from build123d import *

# Parameters (mm, degrees)
F0_W      = 609.6
F0_H      = 762
F1_DEPTH  = 203.2
F2_W      = 76.2
F2_H      = 609.6
F3_DEPTH  = 609.6
F4_W      = 584.2
F4_H      = 76.2
F5_DEPTH  = 101.6
F7_W      = 127
F7_H      = 76.2
F8_DEPTH  = 660.4
F9_W      = 127
F9_H      = 76.2
F10_DEPTH = 660.4
F11_W     = 127
F11_H     = 76.2
F13_DEPTH = 381
F14_DEPTH = 381
F12_W     = 127
F12_H     = 76.2
F15_DEPTH = 381
F16_R     = 25.4
F17_DEPTH = 88.9
F19_R     = 317.5
F20_DEPTH = 50.8


with BuildPart() as f1:
    # F0 (on Front) → F1 (new body)
    with BuildSketch(Plane.XZ):
        with Locations((12.1244145464, 0)):
            Rectangle(F0_W, F0_H)
    extrude(amount=F1_DEPTH)

    # F2 (on face) → F3 (cut)
    with BuildSketch(Plane(origin=(-292.6755854536, 0, 0), x_dir=(0, -1, 0), z_dir=(-1, 0, 0))):
        with Locations((152.4, -76.2)):
            Rectangle(F2_W, F2_H)
    extrude(amount=-F3_DEPTH, mode=Mode.SUBTRACT)

    # F4 (on face) → F5 (cut)
    with BuildSketch(Plane.XY.offset(381)):
        with Locations((12.1244145464, -152.4)):
            Rectangle(F4_W, F4_H)
    extrude(amount=-F5_DEPTH, mode=Mode.SUBTRACT)

    # F7 (on face) → F8 (cut)
    with BuildSketch(Plane.XY.offset(381)):
        with Locations((-216.4755854536, -50.8)):
            Rectangle(F7_W, F7_H)
    extrude(amount=-F8_DEPTH, mode=Mode.SUBTRACT)

    # F9 (on face) → F10 (cut)
    with BuildSketch(Plane.XY.offset(381)):
        with Locations((-64.0755854536, -50.8)):
            Rectangle(F9_W, F9_H)
    extrude(amount=-F10_DEPTH, mode=Mode.SUBTRACT)

    # F11 (on face) → F13 (cut)
    with BuildSketch(Plane.XY.offset(381)):
        with Locations((88.3244145464, -50.8)):
            Rectangle(F11_W, F11_H)
    extrude(amount=-F13_DEPTH, mode=Mode.SUBTRACT)

    # F11 (on face) → F14 (cut)
    with BuildSketch(Plane.XY.offset(381)):
        with Locations((88.3244145464, -50.8)):
            Rectangle(F11_W, F11_H)
    extrude(amount=-F14_DEPTH, mode=Mode.SUBTRACT)

    # F12 (on face) → F15 (cut)
    with BuildSketch(Plane.XY.offset(381)):
        with Locations((240.7244145464, -50.8)):
            Rectangle(F12_W, F12_H)
    extrude(amount=-F15_DEPTH, mode=Mode.SUBTRACT)

    # F16 (on face) → F17 (join)
    with BuildSketch(Plane.XZ.offset(203.2)):
        with Locations((12.1244145464, -114.3)):
            Circle(F16_R)
    extrude(amount=-F17_DEPTH)

    # F19 (on offset) → F20 (join)
    with BuildSketch(Plane.XZ.offset(127)):
        with Locations((12.1244145464, -139.7)):
            Circle(F19_R)
    extrude(amount=F20_DEPTH)


solid = f1.part
Input: part model. Units: mm. Frame: model coordinates. A direction names the side the tool comes from. Coordinates: 2 decimals unless noted, no trailing zeros. Loops run counter-clockwise (first coordinate to the right, second up) from the corner with the lowest first, then second, coordinate; pieces in that order, holes last.
(1) First-contact query: pin 1 Ø4 at (x, z) = (-234.5, 177) entering from +Y; pin 2 Ø10 at (x, y) = (-116.5, -51.5) entering from -Z; pin 3 Ø23 at (y, z) = (-58.5, 41) entering from +X; pin 4 Ø1.5 at (x, y) = (-232.5, -121.5) entering from +Z. Flat tips, straight axial feed; report the tip coordinate or a pass-through.
(2) Section A-A on x = 268. Return the cut outline in (y, z).
(3) Section B-B on z = -294. Return the cut outline in (x, y), then the cut area to 3 significant figures.
(4) Pull-direction query (Y, two-part tool) for faces 5 (the face through (316.924, -78, 79)), 6 (the face through (-65, -50, -279.4)); classes: released by +Y, released by -Y, zero draft, split by the parting line, or undercut.
(5) Section C-C on y = -150. Return the cut outline in (x, z).
(6) Section D-D on z = 305. Return the cut outline in (x, y), then the cut area to 3 significant figures.
(7) Set-up query: faces 1 (the face through (24.824, -51, 193)), 2 (the face through (314.963, -152.044, -44.332)), 3 (the face through (8, -152, 228.6)), 4 (the face through (8, -56, -381)). Return all of +Z, -Z, +X, -X, +Y, -Y with unobstructed straight access to the full face (end or side cutting, diameter ignored); none if empty.
(8) Material intervals for probe 1 along Y at (x, z) = (-39, -68); probe 2 along Y at (x, z) = (-78, -378); probe 3 along X at (y, z) = (-30.5, 63), sorted ascending.
Data:
1. pin 1: stops at y = 0
1. pin 2: stops at z = -381
1. pin 3: stops at x = 316.92
1. pin 4: stops at z = 279.4
2. outline: (-203.2, -381) - (-190.5, -381) - (-190.5, 228.6) - (-114.3, 228.6) - (-114.3, -381) - (0, -381) - (0, 381) - (-12.7, 381) - (-12.7, 0) - (-88.9, 0) - (-88.9, 381) - (-114.3, 381) - (-114.3, 279.4) - (-190.5, 279.4) - (-190.5, 381) - (-203.2, 381) - close; (-177.8, -327.67) - (-127, -327.67) - (-127, 48.27) - (-177.8, 48.27) - close
3. outline: (-292.68, -203.2) - (316.92, -203.2) - (316.92, -190.5) - (-292.68, -190.5) - close; (-292.68, -114.3) - (316.92, -114.3) - (316.92, 0) - (-292.68, 0) - close; (-265.36, -177.8) - (289.61, -177.8) - (289.61, -127) - (-265.36, -127) - close
3. area: 106,000 mm2
4. face 5: zero draft
4. face 6: undercut
5. outline: circle Ø635 at (12.12, -139.7); (-292.68, 228.6) - (316.92, 228.6) - (316.92, 381) - (304.22, 381) - (304.22, 279.4) - (-279.98, 279.4) - (-279.98, 381) - (-292.68, 381) - close
6. outline: (-292.68, -203.2) - (316.92, -203.2) - (316.92, 0) - (-292.68, 0) - close; hole (-279.98, -190.5) - (304.22, -190.5) - (304.22, -114.3) - (-279.98, -114.3) - close; hole (-279.98, -88.9) - (-152.98, -88.9) - (-152.98, -12.7) - (-279.98, -12.7) - close; hole (-127.58, -88.9) - (-0.58, -88.9) - (-0.58, -12.7) - (-127.58, -12.7) - close; hole (24.82, -88.9) - (151.82, -88.9) - (151.82, -12.7) - (24.82, -12.7) - close; hole (177.22, -88.9) - (304.22, -88.9) - (304.22, -12.7) - (177.22, -12.7) - close
6. area: 40,600 mm2
7. face 1: +Z
7. face 2: none
7. face 3: +X, -X
7. face 4: -Z, +X, -X, +Y
8. probe 1: y = -203.2 to -190.5, -177.8 to -127, -114.3 to -88.9, -12.7 to 0
8. probe 2: y = -203.2 to -190.5, -177.8 to -127, -114.3 to 0
8. probe 3: x = -292.68 to -279.98, -152.98 to -127.58, -0.58 to 24.82, 151.82 to 177.22, 304.22 to 316.92
